from build123d import *

# Parameters (mm, degrees)
SKETCH1_W                 = 139.7
SKETCH1_H                 = 139.7
BOSS_EXTRUDE1_DEPTH       = 6.35
F_4_40_TAPPED_HOLE1_D     = 2.2606
F_4_40_TAPPED_HOLE1_DEPTH = 7.5946
F_4_40_TAPPED_HOLE1_TIP   = 0.679152758
F_4_40_TAPPED_HOLE2_D     = 2.2606
F_4_40_TAPPED_HOLE2_DEPTH = 7.5946
F_4_40_TAPPED_HOLE2_TIP   = 0.679152758
F_4_40_TAPPED_HOLE3_D     = 2.2606
F_4_40_TAPPED_HOLE3_DEPTH = 7.5946
F_4_40_TAPPED_HOLE3_TIP   = 0.679152758
F_4_40_TAPPED_HOLE4_D     = 2.2606
F_4_40_TAPPED_HOLE4_DEPTH = 7.5946
F_4_40_TAPPED_HOLE4_TIP   = 0.679152758
SKETCH11_R                = 19.05
CUT_EXTRUDE1_DEPTH        = 7.35
F_2_56_TAPPED_HOLE1_D     = 1.778
F_2_56_TAPPED_HOLE1_DEPTH = 5.7404
F_2_56_TAPPED_HOLE1_TIP   = 0.53416509
F_2_56_TAPPED_HOLE2_D     = 1.778
F_2_56_TAPPED_HOLE2_DEPTH = 5.7404
F_2_56_TAPPED_HOLE2_TIP   = 0.53416509
F_6_0MM_DOWEL_HOLE1_D     = 6


with BuildPart() as part:
    # Sketch1 → Boss-Extrude1 (new body)
    with BuildSketch(Plane.XY):
        Rectangle(SKETCH1_W, SKETCH1_H)
    extrude(amount=BOSS_EXTRUDE1_DEPTH)

    # #4-40 Tapped Hole1
    with Locations(Plane(origin=(0, 69.85, 0), x_dir=(1, 0, 0), z_dir=(0, 1, 0))):
        with Locations((0, -3.175)):
            Hole(F_4_40_TAPPED_HOLE1_D / 2, depth=F_4_40_TAPPED_HOLE1_DEPTH)
            with Locations((0, 0, -(F_4_40_TAPPED_HOLE1_DEPTH + F_4_40_TAPPED_HOLE1_TIP / 2))):  # 118° drill point
                Cone(0, F_4_40_TAPPED_HOLE1_D / 2, F_4_40_TAPPED_HOLE1_TIP, mode=Mode.SUBTRACT)

    # #4-40 Tapped Hole2
    with Locations(Plane(origin=(69.85, 0, 0), x_dir=(0, 0, -1), z_dir=(1, 0, 0))):
        with Locations((-3.175, 0)):
            Hole(F_4_40_TAPPED_HOLE2_D / 2, depth=F_4_40_TAPPED_HOLE2_DEPTH)
            with Locations((0, 0, -(F_4_40_TAPPED_HOLE2_DEPTH + F_4_40_TAPPED_HOLE2_TIP / 2))):  # 118° drill point
                Cone(0, F_4_40_TAPPED_HOLE2_D / 2, F_4_40_TAPPED_HOLE2_TIP, mode=Mode.SUBTRACT)

    # #4-40 Tapped Hole3
    with Locations(Plane(origin=(0, -69.85, 0), x_dir=(-1, 0, 0), z_dir=(0, -1, 0))):
        with Locations((0, -3.175)):
            Hole(F_4_40_TAPPED_HOLE3_D / 2, depth=F_4_40_TAPPED_HOLE3_DEPTH)
            with Locations((0, 0, -(F_4_40_TAPPED_HOLE3_DEPTH + F_4_40_TAPPED_HOLE3_TIP / 2))):  # 118° drill point
                Cone(0, F_4_40_TAPPED_HOLE3_D / 2, F_4_40_TAPPED_HOLE3_TIP, mode=Mode.SUBTRACT)

    # #4-40 Tapped Hole4
    with Locations(Plane.ZY.offset(69.85)):
        with Locations((3.175, 0)):
            Hole(F_4_40_TAPPED_HOLE4_D / 2, depth=F_4_40_TAPPED_HOLE4_DEPTH)
            with Locations((0, 0, -(F_4_40_TAPPED_HOLE4_DEPTH + F_4_40_TAPPED_HOLE4_TIP / 2))):  # 118° drill point
                Cone(0, F_4_40_TAPPED_HOLE4_D / 2, F_4_40_TAPPED_HOLE4_TIP, mode=Mode.SUBTRACT)

    # Sketch11 → Cut-Extrude1 (cut, through all)
    with BuildSketch(Plane(origin=(0, 0, 0), x_dir=(-1, 0, 0), z_dir=(0, 0, -1))):
        with Locations((-44.45, -31.75)):
            Circle(SKETCH11_R)
    extrude(amount=-CUT_EXTRUDE1_DEPTH, mode=Mode.SUBTRACT)

    # #2-56 Tapped Hole1
    with Locations(Plane.XY.offset(6.35)):
        with Locations((-65.786, 65.786), (26.514, 65.786), (-65.786, 13.486), (26.514, 13.486), (-65.786, 3.486), (26.514, 3.486), (-65.786, -48.814), (26.514, -48.814)):
            Hole(F_2_56_TAPPED_HOLE1_D / 2, depth=F_2_56_TAPPED_HOLE1_DEPTH)
            with Locations((0, 0, -(F_2_56_TAPPED_HOLE1_DEPTH + F_2_56_TAPPED_HOLE1_TIP / 2))):  # 118° drill point
                Cone(0, F_2_56_TAPPED_HOLE1_D / 2, F_2_56_TAPPED_HOLE1_TIP, mode=Mode.SUBTRACT)

    # #2-56 Tapped Hole2
    with Locations(Plane(origin=(0, 0, 0), x_dir=(-1, 0, 0), z_dir=(0, 0, -1))):
        with Locations((44.45, 44.45), (44.45, -24.13), (-24.13, -24.13), (-24.13, 44.45)):
            Hole(F_2_56_TAPPED_HOLE2_D / 2, depth=F_2_56_TAPPED_HOLE2_DEPTH)
            with Locations((0, 0, -(F_2_56_TAPPED_HOLE2_DEPTH + F_2_56_TAPPED_HOLE2_TIP / 2))):  # 118° drill point
                Cone(0, F_2_56_TAPPED_HOLE2_D / 2, F_2_56_TAPPED_HOLE2_TIP, mode=Mode.SUBTRACT)

    # Ø6.0mm Dowel Hole1 (through all)
    with Locations(Plane.XY.offset(6.35)):
        with Locations((-57.15, -61.214), (-44.45, -61.214), (-31.75, -61.214), (-19.05, -61.214), (-6.35, -61.214), (6.35, -61.214)):
            Hole(F_6_0MM_DOWEL_HOLE1_D / 2)


solid = part.part
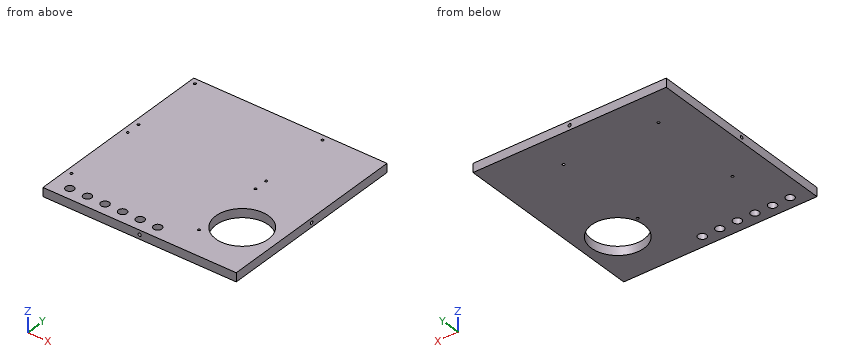
Verification items for the finished model (mm, model axes). Coordinates: 2 decimals unless noted, no trailing zeros. Order: outer loops, then holes, each group sorted by start corner. A loop starts at its lowest first (then second) coordinate and runs counter-clockwise, first axis right, second up.
1. Sectioned sample at A-A, the plane x = 44.45. Record the cut outline in (y, z), and give its area (3 significant figures).
Results found:
outline: (-69.85, 0) - (-50.8, 0) - (-50.8, 6.35) - (-69.85, 6.35) - close; (-12.7, 0) - (69.85, 0) - (69.85, 6.35) - (-12.7, 6.35) - close
area: 645 mm2
2. Sectioned sample at B-B, the plane y = -31.75. Record the cut outline in (x, z), and give its area (3 significant figures).
Results found:
outline: (-69.85, 0) - (25.4, 0) - (25.4, 6.35) - (-69.85, 6.35) - close; (63.5, 0) - (69.85, 0) - (69.85, 6.35) - (63.5, 6.35) - close
area: 645 mm2
3. Scan lines: line 1 (X direction, y = -48.5, z = 1.5); line 2 (Z direction, x = -64, y = 0); line 3 (Y direction, x = -44.45, z = 2.7). Record each from-to range of solid material in increasing order.
Results found:
line 1: x = -69.85 to -66.62, -64.95 to 25.68, 27.35 to 35.38, 53.52 to 69.85
line 2: z = 0 to 2.04, 4.31 to 6.35
line 3: y = -69.85 to -64.21, -58.21 to -25.02, -23.24 to 43.56, 45.34 to 69.85
4. Go/stop test with flat-tipped pins: pin 1 Ø1.6 at (x, y) = (-65.786, 65.786) entering from +Z; pin 2 Ø1.4 at (x, y) = (24.13, -24.13) entering from -Z; pin 3 Ø1.8 at (y, z) = (0, 3.175) entering from +X. Record where each tip stops, or that it passes through.
Results found:
pin 1: stops at z = 0.56
pin 2: stops at z = 5.85
pin 3: stops at x = 62.12
